```python
from build123d import *

# Parameters (mm, degrees)
CHAMFER1_SIZE      = 0.5
SKETCH2_W          = 1
SKETCH2_H          = 2
CUT_EXTRUDE1_DEPTH = 5


with BuildPart() as part:
    # Sketch1 → Revolve1 (revolve)
    with BuildSketch(Plane.XY, mode=Mode.PRIVATE) as revolve1_sk:
        Polygon((0, 0), (3.5, 6.062177826), (3.5, 12), (5, 12), (5, 16), (0, 16), align=None)
    revolve(revolve1_sk.sketch.rotate(Axis((0, 16, 0), (0, -1, 0)), 180), axis=Axis((0, 16, 0), (0, -1, 0)))

    # Chamfer1
    chamfer1_edges = [part.edges().sort_by_distance(p)[0] for p in [
        (5, 16, 0),
        (3.5, 12, 0),
    ]]
    chamfer(chamfer1_edges, length=CHAMFER1_SIZE)

    # Sketch2 → Cut-Extrude1 (cut, symmetric)
    with BuildSketch(Plane.XY):
        with Locations((0, 16)):
            Rectangle(SKETCH2_W, SKETCH2_H)
    extrude(amount=CUT_EXTRUDE1_DEPTH, both=True, mode=Mode.SUBTRACT)


solid = part.part
```
The model under review builds one solid part; all positions refer to its coordinate system, in mm. A direction names the side the tool comes from. Give positions to 0.01 mm unless a question says otherwise; leave off trailing zeros. Order: outer loops, then holes, each group sorted by start corner. A loop starts at its lowest first (then second) coordinate and runs counter-clockwise, first axis right, second up. Notation, with made-up numbers: (71.5, 13) - (127.5, 13) arc R21 cw to (127.5, 18) - close; hole circle Ø8 at (48.5, 76.5). An arc over 180 degrees is marked (long way). Use CSV: the item, a comma, the result in double quotes. Start each with the question number.
Q1. To check wall thickness, follow line 1 along Z through (x, y) = (0, 10.25); line 2 along Y through (x, z) = (0.25, 4.75); line 3 along Z through (x, y) = (0.5, 14.25). State the ranges of each line that lie inside material, in increasing order. Write a range as [from, to].
Q2. We need section B-B, the plane y = 1.75. Write out the cut boundary in (x, z).
Q3. Tool access review of faces 1 (the flat face through (0, 15, 0)), 2 (the conical face through (4.634, 15.865, -0.095)): name each direction out of +Z, -Z, +X, -X, +Y, -Y from which nothing blocks a thin tool from reaching the whole face with its end or side.
Q4. We need section A-A, the plane y = 9.5. Write out the cut boundary in (x, z), and give its area (3 significant figures).
Q5. The part is to be moulded in two halves that separate along X. For faces 3 (the cylindrical face through (-3.233, 8.819, 1.341)), 4 (the flat face through (0.5, 15.5, 0.1)), 5 (the flat face through (-2, 16, 0)), 6 (the flat face through (-0.5, 15.5, 0.1)), say which applies: +X half, -X half, draft (parallel to the pull), parting line (faces both ways), or undercut.
Q6. Clearance check with flat-ended pins moving along their axes: pin 1 Ø3 at (y, z) = (4, -2) entering from -X; pin 2 Ø0.5 at (y, z) = (15.5, -1.5) entering from -X; pin 3 Ø1.5 at (y, z) = (7, -2.5) entering from -X. State where each tip first meets the part, or that it passes through.
Outcome:
1,line 1,"z = [-3.5, 3.5]"
1,line 2,"y = [12, 15]"
1,line 3,"z = [-4.97, 4.97]"
2,outline,"circle Ø2.02 at (0, 0)"
3,face 1,"+Z, -Z, +Y"
3,face 2,"+X, +Y"
4,outline,"circle Ø7 at (0, 0)"
4,area,"38.5 mm^2"
5,face 3,"parting line"
5,face 4,"undercut"
5,face 5,"draft"
5,face 6,"undercut"
6,pin 1,"stops at x = -2.8"
6,pin 2,"stops at x = -4.84"
6,pin 3,"stops at x = -3.03"
